Verification items for the finished model (mm, model axes). A direction names the side the tool comes from. Coordinates: 2 decimals unless noted, no trailing zeros. Write each loop counter-clockwise with the first axis right and the second up, starting at its lowest first coordinate (ties: lowest second). Pieces come first, ordered by that corner, then holes. Notation, with made-up numbers: (30.5, -14.5) -> (71.5, -14.5) arc R26 ccw to (71.5, 6.5) -> close; hole circle Ø2 at (-13.75, 61.25). An arc over 180 degrees is marked (long way). Answer in a Markdown table with one row per item.
Autodesk Inventor part; units mm, degrees
ref_plane "YZ Plane" through (0, 0, 0) normal (1, 0, 0) x (0, 1, 0)
ref_plane "XZ Plane" through (0, 0, 0) normal (0, 1, 0) x (-1, 0, 0)
ref_plane "XY Plane" through (0, 0, 0) normal (0, 0, 1) x (1, 0, 0)
sketch "スケッチ1" plane through (0, 0, 0) normal (0, 0, 1) x (1, 0, 0)
  circle A0 centre (0, 0) radius 9.3
  circle A1 centre (0, 0) radius 0.75
  dimension "d0" = 18.6
  dimension "d1" = 1.5
extrude "押し出し1" add sketch "スケッチ1" along normal blind 1
sketch "スケッチ2" plane through (0, 0, 1) normal (0, 0, 1) x (1, 0, 0)
  circle A0 centre (0, 0) radius 0.75
  circle A1 centre (0, 0) radius 9.3
  circle A2 centre (0, 0) radius 6.5
  dimension "d4" = 13
extrude "押し出し2" add sketch "スケッチ2" along normal blind 1 contours A1
sketch "スケッチ3" plane through (0, 0, 0) normal (0, 0, -1) x (-1, 0, 0)
  circle A0 centre (0, 0) radius 6.5
  circle A1 centre (0, 0) radius 0.75
  circle A2 centre (0, 0) radius 9.3
extrude "押し出し3" add sketch "スケッチ3" along normal blind 1 contours A2
chamfer "面取り1" distance 0.6 angle 45 2 edges at (6.5, 0, 0) (-6.5, 0, 1)
properties part number "RescueKitThrow_springholder"
1. Section check C-C, the plane z = 0.35. Record the boundary of the cut face in (x, y).
Geometry says:
| item | result |
|---|---|
| outline | circle Ø18.6 at (0, 0); hole circle Ø1.5 at (0, 0) |
2. Depth check by flat-ended pin: P1, Ø10.5, axis at x = 0, y = 0, coming from the -Z side; P2, Ø10.5, axis at x = 0, y = 0, coming from the +Z side; P3, Ø0.9, axis at x = 0, y = 0, coming from the +Z side; P4, Ø1.5, axis at x = 2, z = 0, coming from the -Y side. Enter the tip coordinate at first touch or a pass-through.
Geometry says:
| item | result |
|---|---|
| P1 | z = 0 |
| P2 | z = 1 |
| P3 | through |
| P4 | y = -9.22 |
3. Tool access check on faces 1 (the flat face through (-2.2, 6.3, 2)), 2 (the cylindrical face through (5.158, 3.955, -0.797)), 3 (the cylindrical face through (-5.158, 3.955, 1.797)). Record the directions out of +Z, -Z, +X, -X, +Y, -Y that give a thin tool (end or side, any length) a straight path to the whole face; none if there is none.
Geometry says:
| item | result |
|---|---|
| face 1 | +Z, +X, -X, +Y, -Y |
| face 2 | -Z |
| face 3 | +Z |
4. Mould release check, pull along X, two halves, no side actions. Record for faces 4 (the flat face through (1, 0, 0)), 5 (the flat face through (2.2, 6.3, -1)): released by +X, released by -X, zero draft, split by the parting line, or undercut.
Geometry says:
| item | result |
|---|---|
| face 4 | undercut |
| face 5 | zero draft |
5. Section check A-A, the plane y = 0. Record the boundary of the cut face in (x, z), plus the area to 3 significant figures.
Geometry says:
| item | result |
|---|---|
| outline | (-9.3, -1) -> (-6.5, -1) -> (-6.5, -0.6) -> (-5.9, 0) -> (-0.75, 0) -> (-0.75, 1) -> (-5.9, 1) -> (-6.5, 1.6) -> (-6.5, 2) -> (-9.3, 2) -> close; (0.75, 0) -> (5.9, 0) -> (6.5, -0.6) -> (6.5, -1) -> (9.3, -1) -> (9.3, 2) -> (6.5, 2) -> (6.5, 1.6) -> (5.9, 1) -> (0.75, 1) -> close |
| area | 29.0 mm^2 |
6. Section check D-D, the plane y = 7. Record the boundary of the cut face in (x, z).
Geometry says:
| item | result |
|---|---|
| outline | (-6.12, -1) -> (6.12, -1) -> (6.12, 2) -> (-6.12, 2) -> close |
7. Thickness scan on line 1 (Y direction, x = 0, z = 1.85); line 2 (Z direction, x = -3.75, y = 3); line 3 (Y direction, x = 5.5, z = 1.4). Record the ranges inside material, lowest first. Write a range as from..to.
Geometry says:
| item | result |
|---|---|
| line 1 | -9.3..-6.5, 6.5..9.3 |
| line 2 | 0..1 |
| line 3 | -7.5..-3.07, 3.07..7.5 |
